Geometry check sheet. Reference: the model listing, model coordinates, mm. A direction names the side the tool comes from. Coordinates: 2 decimals unless noted, no trailing zeros. Order: outer loops, then holes, each group sorted by start corner. A loop starts at its lowest first (then second) coordinate and runs counter-clockwise, first axis right, second up. Notation, with made-up numbers: (5.5, 35) - (23.5, 35) arc R15 cw to (23.5, 64) - close; hole circle Ø8 at (67.25, -8). An arc over 180 degrees is marked (long way). Use CSV: the item, a comma, the result in double quotes. Start each with the question number.
1) Draft check along X on faces 1 (the flat face through (5, -9, 7.798)), 2 (the flat face through (17.43, -9, 4)), 3 (the cylindrical face through (6.317, -15.615, 3.638)). Enter one of: released by +X, released by -X, zero draft, split by the parting line, or undercut.
2) Sectioned sample at A-A, the plane x = -5. Record the cut outline in (y, z) (3 decimals).
3) Sectioned sample at D-D, the plane x = 14. Record the cut outline in (y, z) (3 decimals), and give its area (3 significant figures).
4) Thickness scan on probe 1 along Z at (x, y) = (-12, -1.25); probe 2 along X at (y, z) = (-13, -11); probe 3 along X at (y, z) = (-7.25, -7). Record the ranges inside material, lowest first. Write a range as [from, to].
5) Tool access check on faces 4 (the flat face through (4.37, -13.62, -16.42)), 5 (the conical face through (0.26, -10.04, -1.94)), 6 (the flat face through (30.13, -9, 1)), 7 (the cylindrical face through (-1.887, -7.005, 1.741)), 8 (the cylindrical face through (-15.907, -3.34, 3.708)). Record the directions out of +Z, -Z, +X, -X, +Y, -Y that give a thin tool (end or side, any length) a straight path to the whole face; none if there is none.
6) Sectioned sample at C-C, the plane z = 3. Record the cut outline in (x, y), and give its area (3 significant figures).
7) Depth check by flat-ended pin: P1, Ø10, axis at y = -15, z = -24, coming from the +X side; P2, Ø2, axis at x = -1, y = -4.5, coming from the -Z side; P3, Ø2, axis at y = -10, z = -22.5, coming from the +X side. Enter the tip coordinate at first touch or a pass-through.
8) Sectioned sample at B-B, the plane y = -16.25. Record the cut outline in (x, z) (1 decimal), and give its area (3 significant figures).
from build123d import *

# Parameters (mm, degrees)
F1_DEPTH = 19.05
F3_R     = 3.175
F4_DEPTH = 38.1
F6_DEPTH = 19.05
F8_D     = 8.8
F8_DEPTH = 12.7
F8_TIP   = 2.6437867237


with BuildPart() as f1:
    # F0 (on Front) → F1 (new body)
    with BuildSketch(Plane.XZ):
        Polygon((-20.6700884257, 7.7979226127), (-20.6700884257, -27.7620773873), (30.1299115743, -4.7548310105), (30.1299115743, 7.7979226127), align=None)
    extrude(amount=F1_DEPTH)

    # F3 (on face) → F4 (cut)
    with BuildSketch(Plane(origin=(-20.6700884257, 0, 0), x_dir=(0, -1, 0), z_dir=(-1, 0, 0))):
        with Locations((9.525, 3.6731153582)):
            Circle(F3_R)
    extrude(amount=-F4_DEPTH, mode=Mode.SUBTRACT)

    # F5 (on face) → F6 (cut, through all)
    with BuildSketch(Plane.XZ):
        with BuildLine():
            ThreePointArc((4.7299115743, 2.0856153582), (6.3174115743, 3.6731153582), (4.7299115743, 5.2606153582))
            Line((4.7299115743, 5.2606153582), (-14.3200884257, 5.2606153582))
            ThreePointArc((-14.3200884257, 5.2606153582), (-15.9075884257, 3.6731153582), (-14.3200884257, 2.0856153582))
            Line((-14.3200884257, 2.0856153582), (4.7299115743, 2.0856153582))
        make_face()
    extrude(amount=F6_DEPTH, mode=Mode.SUBTRACT)

    # F8
    with Locations(Plane(origin=(6.9151919719, 0, -15.2687438739), x_dir=(0.9109307781, 0, 0.4125592292), z_dir=(0.4125592292, 0, -0.9109307781))):
        with Locations((0, 9.525)):
            Hole(F8_D / 2, depth=F8_DEPTH)
            with Locations((0, 0, -(F8_DEPTH + F8_TIP / 2))):  # 118° drill point
                Cone(0, F8_D / 2, F8_TIP, mode=Mode.SUBTRACT)


solid = f1.part
Evaluation:
1,face 1,"zero draft"
1,face 2,"released by -X"
1,face 3,"undercut"
2,outline,"(-19.05, -20.665) - (0, -20.665) - (0, 2.086) - (-6.775, 2.086) arc R3.175 cw to (-12.275, 2.086) - (-19.05, 2.086) - close; (-19.05, 5.261) - (-12.275, 5.261) arc R3.175 cw to (-6.775, 5.261) - (0, 5.261) - (0, 7.798) - (-19.05, 7.798) - close"
3,outline,"(-19.05, -12.06) - (0, -12.06) - (0, 7.798) - (-19.05, 7.798) - close; hole circle Ø6.35 at (-9.525, 3.673)"
3,area,"347 mm²"
4,probe 1,"[-23.84, 2.09], [5.26, 7.8]"
4,probe 2,"[-20.67, 2.02], [7.94, 16.34]"
4,probe 3,"[-20.67, -0.96], [7.3, 25.17]"
5,face 4,"-Z, +X, +Y, -Y"
5,face 5,"none"
5,face 6,"+Z, -Z, +X, +Y, -Y"
5,face 7,"-X"
5,face 8,"+Y, -Y"
6,outline,"(-20.67, -19.05) - (-15.76, -19.05) - (-15.76, -12.63) - (-20.67, -12.63) - close; (-20.67, -6.42) - (-15.76, -6.42) - (-15.76, 0) - (-20.67, 0) - close; (6.17, -19.05) - (30.13, -19.05) - (30.13, 0) - (6.17, 0) - (6.17, -6.42) - (17.43, -6.42) - (17.43, -12.63) - (6.17, -12.63) - close"
6,area,"450 mm²"
7,P1,"x = -1.32"
7,P2,"z = -19.31"
7,P3,"x = -6.84"
8,outline,"(-20.7, -27.8) - (30.1, -4.8) - (30.1, 7.8) - (-20.7, 7.8) - close; hole (-14.3, 2.1) - (4.7, 2.1) arc R1.6 ccw to (4.7, 5.3) - (-14.3, 5.3) arc R1.6 ccw to start"
8,area,"1,150 mm²"
